Design review of the part shown in the three views and the two pictorial views. Dimensions are in mm from the part's minimum x, y and z. A direction names the side the tool comes from. Round coordinates to 2 decimals unless told otherwise and drop trailing zeros. Loops run counter-clockwise (first coordinate to the right, second up) from the corner with the lowest first, then second, coordinate; pieces in that order, holes last. Notation, with made-up numbers: (82.5, 24) -> (102.5, 24) arc R9 ccw to (102.5, 30) -> close; hole circle Ø8 at (33, 3). An arc over 180 degrees is marked (long way). Write each question's results on one line, items separated by ' | '. Start each with the question number.
Item 1: We need section A-A (x = 34.5). Give the boundary of the cut face in (y, z), and give its area (3 significant figures).
Item 2: We need section B-B (y = 104.5). Give the boundary of the cut face in (x, z), and give its area (3 significant figures).
Item 3: For L1, parallel to Z at x = 24, y = 36; L2, parallel to X at y = 175, z = 113; L3, parallel to X at y = 84.5, z = 11, list the stretches that pass through material, from the lowest coordinate up. Write a range as from..to.
Item 4: Tool access review of the marked faces 1 and 2: name each direction out of +Z, -Z, +X, -X, +Y, -Y from which nothing blocks a thin tool from reaching the whole face with its end or side.
Item 5: We need section C-C (z = 79.5). Give the boundary of the cut face in (x, y), and give its area (3 significant figures).
Item 6: Mouldability with a two-part tool opening along Z and no side actions: class the marked faces 3, 4 and 5 as pulls with the +Z half, pulls with the -Z half, needs draft (parallel to the pull), parting line crosses it, or undercut.
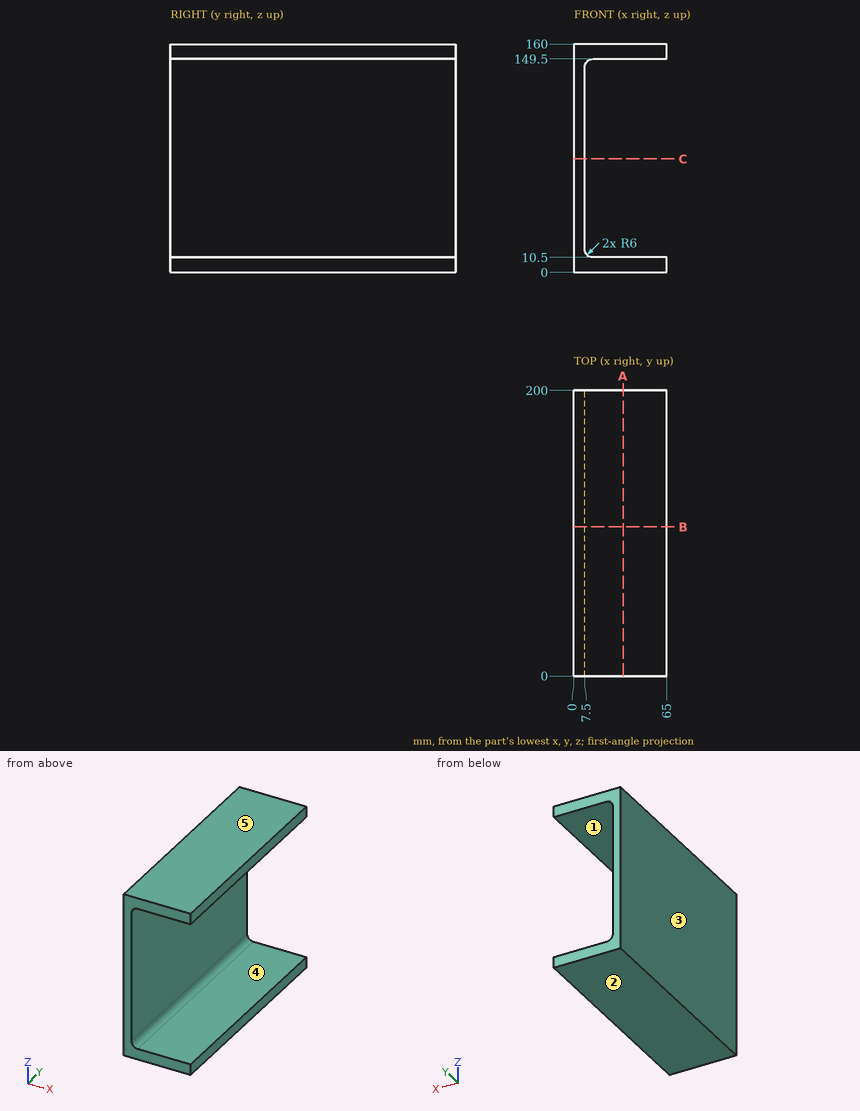
Here are the results:
1) outline: (0, 0) -> (200, 0) -> (200, 10.5) -> (0, 10.5) -> close; (0, 149.5) -> (200, 149.5) -> (200, 160) -> (0, 160) -> close | area: 4,200 mm2
2) outline: (0, 0) -> (65, 0) -> (65, 10.5) -> (13.5, 10.5) arc R6 cw to (7.5, 16.5) -> (7.5, 143.5) arc R6 cw to (13.5, 149.5) -> (65, 149.5) -> (65, 160) -> (0, 160) -> close | area: 2,420 mm2
3) L1: z = 0..10.5, 149.5..160 | L2: x = 0..7.5 | L3: x = 0..11.1
4) face 1: +X, +Y, -Y | face 2: -Z, +X, -X, +Y, -Y
5) outline: (0, 0) -> (7.5, 0) -> (7.5, 200) -> (0, 200) -> close | area: 1,500 mm2
6) face 3: needs draft | face 4: undercut | face 5: pulls with the +Z half
